Work out the finished part from the listing and answer in its coordinate system (mm). Face numbers are marked on the shaded views. A direction names the side the tool comes from. Give positions to 0.01 mm unless a question says otherwise; leave off trailing zeros. Order: outer loops, then holes, each group sorted by start corner. A loop starts at its lowest first (then second) coordinate and runs counter-clockwise, first axis right, second up.
```python
from build123d import *

# Parameters (mm, degrees)
SKETCH_1_R          = 11
EXTRUDE_1_DEPTH     = 2
SKETCH_2_R          = 7
EXTRUDE_2_DEPTH     = 8
SKETCH_3_R          = 5
CUT_EXTRUDE_1_DEPTH = 19.493242009
CHAMFER_1_SIZE      = 0.2


with BuildPart() as part:
    # 草图1 → 凸台-拉伸1 (new body)
    with BuildSketch(Plane(origin=(0, 0, 0), x_dir=(0, 0, -1), z_dir=(1, 0, 0))):
        Circle(SKETCH_1_R)
    extrude(amount=EXTRUDE_1_DEPTH)

    # 草图2 → 凸台-拉伸2 (add)
    with BuildSketch(Plane(origin=(2, 0, 0), x_dir=(0, 0, -1), z_dir=(1, 0, 0))):
        Circle(SKETCH_2_R)
    extrude(amount=EXTRUDE_2_DEPTH)

    # 草图3 → 切除-拉伸1 (cut, through all)
    with BuildSketch(Plane(origin=(10, 0, 0), x_dir=(0, 0, -1), z_dir=(1, 0, 0))):
        Circle(SKETCH_3_R)
    extrude(amount=-CUT_EXTRUDE_1_DEPTH, mode=Mode.SUBTRACT)

    # 倒角1
    chamfer_1_edges = [part.edges().sort_by_distance(p)[0] for p in [
        (0, 0, 5),
        (10, 0, 5),
        (0, 0, 11),
        (2, 0, 11),
        (10, 0, 7),
    ]]
    chamfer(chamfer_1_edges, length=CHAMFER_1_SIZE)


solid = part.part
```
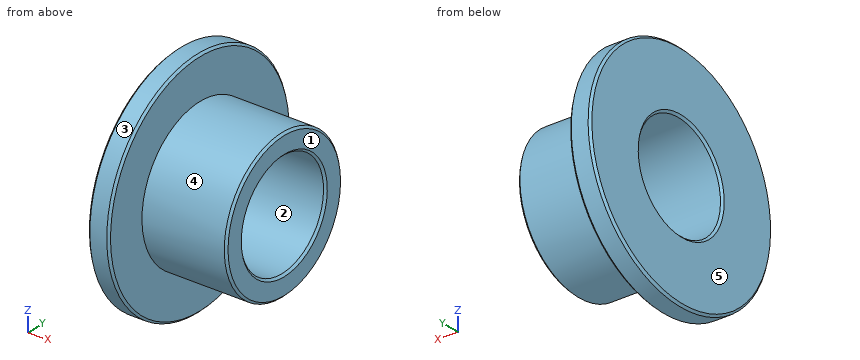
1. Which of the six approach directions +Z, -Z, +X, -X, +Y, -Y give full straight-line access (tool end or side, diameter ignored) to the marked faces 4 and 5?
Findings below:
face 4: +X
face 5: +Z, -Z, -X, +Y, -Y
2. The part is cut by section C-C (x = 8). Write down the section's boundary in (y, z), then the cut area to 3 significant figures.
Findings below:
outline: circle Ø14 at (0, 0); hole circle Ø10 at (0, 0)
area: 75.4 mm2
3. Straight lines are drawn through the part: probe 1 along Y at (x, z) = (6.25, 0); probe 2 along X at (y, z) = (2.5, 8.5); probe 3 along Y at (x, z) = (5, -1.5). For each, find the intervals that lie inside material, in ascending order.
Findings below:
probe 1: y = -7 to -5, 5 to 7
probe 2: x = 0 to 2
probe 3: y = -6.84 to -4.77, 4.77 to 6.84
4. The mould has two halves that part along Y. Classify the marked faces 1, 2 and 3: pulls with the +Y half, pulls with the -Y half, needs draft (parallel to the pull), parting line crosses it, or undercut.
Findings below:
face 1: needs draft
face 2: undercut
face 3: parting line crosses it
5. Given P1, Ø6, axis at y = -2, z = 0.5, coming from the +X side; P2, Ø6, axis at y = -8.5, z = 7, coming from the +X side; P3, Ø2, axis at x = 7.5, y = 0.5, coming from the -Z side, each flat-ended and moving along its own axis, determine where each tip first touches the part or whether it passes through.
Findings below:
P1: stops at x = 9.86
P2: stops at x = 2
P3: stops at z = -7
6. The part is cut by section A-A (y = 0). Write down the section's boundary in (x, z), then the cut area to 3 significant figures.
Findings below:
outline: (0, -10.8) - (0.2, -11) - (1.8, -11) - (2, -10.8) - (2, -7) - (9.8, -7) - (10, -6.8) - (10, -5.2) - (9.8, -5) - (0.2, -5) - (0, -5.2) - close; (0, 5.2) - (0.2, 5) - (9.8, 5) - (10, 5.2) - (10, 6.8) - (9.8, 7) - (2, 7) - (2, 10.8) - (1.8, 11) - (0.2, 11) - (0, 10.8) - close
area: 55.8 mm2
